Source: three-view drawing plus pictorial views. Frame: mm from the lowest corner of the part. A direction names the side the tool comes from. Give positions to 0.01 mm unless a question says otherwise; leave off trailing zeros. Write each loop counter-clockwise with the first axis right and the second up, starting at its lowest first coordinate (ties: lowest second). Pieces come first, ordered by that corner, then holes. Notation, with made-up numbers: M -5,6 L 48,6 A29 cw 48,27 Z; hole C 39,22 d3. An arc over 180 degrees is marked long. Return JSON: item names as keys, results as strings.
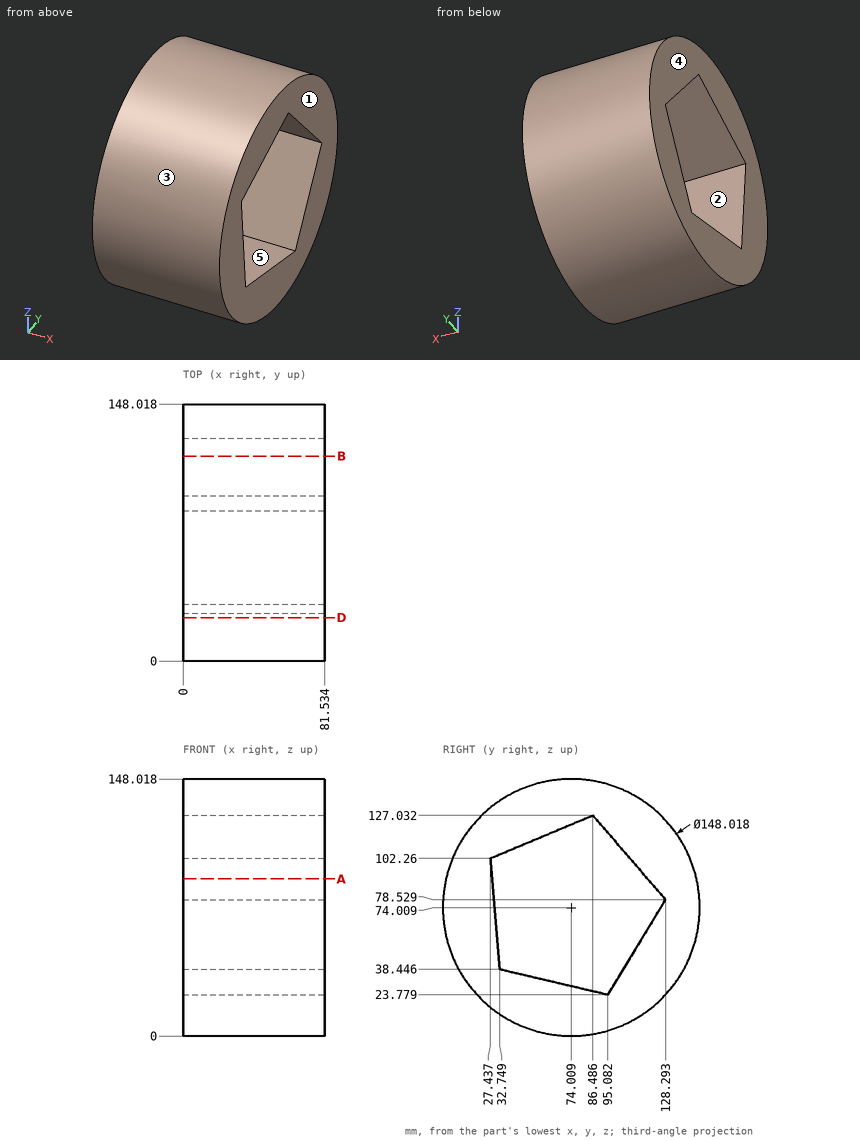
1) Line query: line 1 (Y direction, x = 78, z = 92); line 2 (Y direction, x = 15, z = 49) (1 decimal); line 3 (Z direction, x = 29.5, y = 55.5) (1 decimal). Output: solid intervals per line, ascending. Write a range as [from, to].
Numbers:
{"line 1": "y = [2.22, 28.29], [116.68, 145.8]", "line 2": "y = [4.4, 31.9], [110.4, 143.7]", "line 3": "z = [2.4, 33.1], [114, 145.7]"}
2) Cut plane A-A, the plane z = 90.5. Return the cut outline in (x, y) (1 decimal).
Numbers:
{"outline": "M 0,1.9 L 81.5,1.9 L 81.5,28.4 L 0,28.4 Z; M 0,118 L 81.5,118 L 81.5,146.2 L 0,146.2 Z"}
3) Cut plane B-B, the plane y = 118. Return the cut outline in (x, z) (1 decimal).
Numbers:
{"outline": "M 0,14.5 L 81.5,14.5 L 81.5,61.6 L 0,61.6 Z; M 0,90.5 L 81.5,90.5 L 81.5,133.5 L 0,133.5 Z"}
4) Draft query along Y for the marked faces 1, 2 and 3. Return one class per face: released by +Y, released by -Y, zero draft, split by the parting line, or undercut.
Numbers:
{"face 1": "zero draft", "face 2": "undercut", "face 3": "split by the parting line"}
5) Contact query for flat-ended pins moving along their axis: pin 1 Ø5 at (x, y) = (43.5, 98.5) entering from +Z (1 decimal); pin 2 Ø2 at (x, y) = (55.5, 104) entering from +Z (1 decimal); pin 3 Ø4 at (x, z) = (11, 104) entering from +Y. Output: stop coordinate, or through.
Numbers:
{"pin 1": "stops at z = 144.7", "pin 2": "stops at z = 142.1", "pin 3": "stops at y = 142.52"}
6) Set-up query: the marked faces 4 and 5. Return all of +Z, -Z, +X, -X, +Y, -Y with unobstructed straight access to the full face (end or side cutting, diameter ignored); none if empty.
Numbers:
{"face 4": "+Z, -Z, -X, +Y, -Y", "face 5": "+X, -X"}
7) Cut plane D-D, the plane y = 25. Return the cut outline in (x, z) (1 decimal), then the cut area to 3 significant figures.
Numbers:
{"outline": "M 0,18.6 L 81.5,18.6 L 81.5,129.5 L 0,129.5 Z", "area": "9,040 mm²"}
